```python
from build123d import *

# Parameters (mm, degrees)
SKICA1_W                 = 25.8
SKICA1_H                 = 21.7
SKICA1_R                 = 1.6
P_IDAT_VYSUNUT_M1_DEPTH  = 4
SKICA2_W                 = 4
SKICA2_H                 = 21.7
P_IDAT_VYSUNUT_M2_DEPTH  = 4
SKICA4_R                 = 5.25
SKICA4_R_2               = 1.6
P_IDAT_VYSUNUT_M3_DEPTH  = 21.7
ZKOSEN_1_SIZE            = 7
SKICA5_R                 = 5
ODEBRAT_VYSUNUT_M1_DEPTH = 3


with BuildPart() as part:
    # Skica1 → Přidat vysunutím1 (new body)
    with BuildSketch(Plane.XY):
        with Locations((3.311981452, -9.09140889)):
            Rectangle(SKICA1_W, SKICA1_H)
        with Locations((-6.688018548, -1.59140889)):
            Circle(SKICA1_R, mode=Mode.SUBTRACT)
        with Locations((13.311981452, -1.59140889)):
            Circle(SKICA1_R, mode=Mode.SUBTRACT)
        with Locations((13.311981452, -16.59140889)):
            Circle(SKICA1_R, mode=Mode.SUBTRACT)
        with Locations((-6.688018548, -16.59140889)):
            Circle(SKICA1_R, mode=Mode.SUBTRACT)
    extrude(amount=P_IDAT_VYSUNUT_M1_DEPTH)

    # Skica2 → Přidat vysunutím2 (add)
    with BuildSketch(Plane.ZY.offset(9.588018548)):
        with Locations((2, -9.09140889)):
            Rectangle(SKICA2_W, SKICA2_H)
    extrude(amount=P_IDAT_VYSUNUT_M2_DEPTH)

    # Skica4 → Přidat vysunutím3 (add)
    with BuildSketch(Plane(origin=(0, 1.75859111, 0), x_dir=(1, 0, 0), z_dir=(0, 1, 0))):
        Polygon((-13.588018548, -4), (-13.588018548, 0), (-10.783404097, 0), (-15.62281297, 4.500209586), (-20.589130875, 15.483860416), (-20.589130875, 33.262325999), (-20.589130875, 58.037674001), (-45.99437508, 58.037674001), (-45.99437508, 33.262325999), (-43.640152305, 30.908103223), (-43.640152305, 20.059780683), align=None)
        with Locations(Location((-33.291752977, 45.65, 0), (0, 0, 270))):
            Circle(SKICA4_R, mode=Mode.SUBTRACT)
        with Locations(Location((-39.019164168, 51.235406078, 0), (0, 0, 270))):
            Circle(SKICA4_R_2, mode=Mode.SUBTRACT)
        with Locations(Location((-27.564341787, 40.064593922, 0), (0, 0, 270))):
            Circle(SKICA4_R_2, mode=Mode.SUBTRACT)
    extrude(amount=-P_IDAT_VYSUNUT_M3_DEPTH)

    # Zkosení1
    zkosen_1_edges = [part.edges().sort_by_distance(p)[0] for p in [
        (-45.99437508, -9.09140889, -58.037674001),
    ]]
    chamfer(zkosen_1_edges, length=ZKOSEN_1_SIZE)

    # Skica5 → Odebrat vysunutím1 (cut)
    with BuildSketch(Plane(origin=(-20.589130875, 0, 0), x_dir=(0, 0, -1), z_dir=(1, 0, 0))):
        with Locations((24.263711451, -9.09140889)):
            Circle(SKICA5_R)
        with Locations((45.216218307, -9.09140889)):
            Circle(SKICA5_R)
    extrude(amount=-ODEBRAT_VYSUNUT_M1_DEPTH, mode=Mode.SUBTRACT)


solid = part.part
```
Source: CAD feature listing. Evaluate the final solid. Frame: model axes, mm. A direction names the side the tool comes from. Give positions to 0.01 mm unless a question says otherwise; leave off trailing zeros. Order: outer loops, then holes, each group sorted by start corner. A loop starts at its lowest first (then second) coordinate and runs counter-clockwise, first axis right, second up.
(1) Access query for faces 5 (the face through (3, -9, 0)), 6 (the face through (16.212, -9, 2)), 7 (the face through (-22.068, -7.59, -49.985)), 8 (the face through (-43.64, -9, -26)). Directions: +Z, -Z, +X, -X, +Y, -Y. A direction counts if a zero-diameter tool reaches every point of the face in a straight line with its end or side. Return the directions, or none.
(2) Section query B-B (y = -6). Return the cut outline in (x, z), plus the area to 3 significant figures.
(3) Section query D-D (z = -32). Return the cut outline in (x, y), plus the area to 3 significant figures.
(4) Section query C-C (x = 2.5). Return the cut outline in (y, z).
(5) Material intervals for line 1 along X through (y, z) = (-12.25, -41); line 2 along X through (y, z) = (-11.5, -50.5); line 3 along Z through (x, y) = (10, -10.25), sorted ascending.
(6) Pull-direction query (X, two-part tool) for faces 1 (the face through (-44.83, -8.94, -32.1)), 2 (the face through (-23.589, -9, -45)), 3 (the face through (-27, -19.941, -29)), 4 (the face through (-27.08, -8.94, -38.54)); classes: +X half, -X half, draft (parallel to the pull), parting line (faces both ways), or undercut.
(7) Contact query for flat-ended pins moving along their axis: P1, Ø5, axis at y = -11, z = -25, coming from the +X side; P2, Ø6, axis at y = -12, z = -22.5, coming from the +X side; P3, Ø10, axis at y = -7, z = -12.5, coming from the +X side; P4, Ø10, axis at x = -31.5, z = -6.5, coming from the +Y side. Output: stop coordinate, or through.
(8) Section query A-A (z = -45.65). Return the cut outline in (x, y).
Outcome:
1. face 5: -Z, +X, +Y, -Y
1. face 6: +Z, -Z, +X, +Y, -Y
1. face 7: +X
1. face 8: +Z, -X, +Y, -Y
2. outline: (-45.99, -51.04) - (-38.99, -58.04) - (-20.59, -58.04) - (-20.59, -49.15) - (-23.59, -49.15) - (-23.59, -41.29) - (-20.59, -41.29) - (-20.59, -28.19) - (-23.59, -28.19) - (-23.59, -20.33) - (-20.59, -20.33) - (-20.59, -15.48) - (-15.62, -4.5) - (-10.78, 0) - (16.21, 0) - (16.21, 4) - (-13.59, 4) - (-43.64, -20.06) - (-43.64, -30.91) - (-45.99, -33.26) - close; hole circle Ø3.2 at (-39.02, -51.24); hole circle Ø10.5 at (-33.29, -45.65); hole circle Ø3.2 at (-27.56, -40.06)
2. area: 1,160 mm2
3. outline: (-44.73, -19.94) - (-20.59, -19.94) - (-20.59, 1.76) - (-44.73, 1.76) - close
3. area: 524 mm2
4. outline: (-19.94, 0) - (1.76, 0) - (1.76, 4) - (-19.94, 4) - close
5. line 1: x = -45.99 to -35.73, -30.85 to -28.86, -26.27 to -20.59
5. line 2: x = -45.99 to -40.44, -37.6 to -35.3, -31.28 to -20.59
5. line 3: z = 0 to 4
6. face 1: -X half
6. face 2: +X half
6. face 3: draft
6. face 4: undercut
7. P1: stops at x = -23.59
7. P2: stops at x = -20.59
7. P3: stops at x = -16.98
7. P4: stops at y = 1.76
8. outline: (-45.99, -19.94) - (-38.54, -19.94) - (-38.54, 1.76) - (-45.99, 1.76) - close; (-28.04, -19.94) - (-20.59, -19.94) - (-20.59, -14.07) - (-23.59, -14.07) - (-23.59, -4.11) - (-20.59, -4.11) - (-20.59, 1.76) - (-28.04, 1.76) - close
